Read the model definition and answer for the solid it produces. Units are mm, in the model's axes. A direction names the side the tool comes from. Coordinates: 2 decimals unless noted, no trailing zeros. Loops run counter-clockwise (first coordinate to the right, second up) from the corner with the lowest first, then second, coordinate; pieces in that order, holes last.
from build123d import *

# Parameters (mm, degrees)
SKETCH1_W                 = 201.168
SKETCH1_H                 = 201.168
BOSS_EXTRUDE1_DEPTH       = 1.5875
CUT_EXTRUDE1_REACH        = 144.256
SKETCH2_R                 = 16.5
F_1_4_CLEARANCE_HOLE1_D   = 6.7564
CHAMFER1_SIZE             = 6.35
CUT_EXTRUDE3_REACH        = 144.256
CUT_EXTRUDE4_REACH        = 144.256
CUT_EXTRUDE5_REACH        = 144.256
SKETCH7_W                 = 6.7564
SKETCH7_H                 = 14.478
SKETCH7_W_2               = 14.478
SKETCH7_H_2               = 6.7564
PORT_FOR_POWER_PLUG_REACH = 144.256
SKETCH8_R                 = 6.35


with BuildPart() as part:
    # Sketch1 → Boss-Extrude1 (new body)
    with BuildSketch(Plane.XY):
        Rectangle(SKETCH1_W, SKETCH1_H)
    extrude(amount=BOSS_EXTRUDE1_DEPTH)

    # Sketch2 → Cut-Extrude1 (cut, up to next)
    with BuildSketch(Plane.XY.offset(1.5875), mode=Mode.PRIVATE) as cut_extrude1_sk1:
        with Locations((-49.784, -40.5765)):
            Circle(SKETCH2_R)
    cut_extrude1_tool1 = extrude(cut_extrude1_sk1.sketch, amount=-CUT_EXTRUDE1_REACH, mode=Mode.PRIVATE) & part.part
    # Sketch2 → Cut-Extrude1 (cut, up to next)
    with BuildSketch(Plane.XY.offset(1.5875), mode=Mode.PRIVATE) as cut_extrude1_sk2:
        with Locations((39.4206, -52.284)):
            Circle(SKETCH2_R)
    cut_extrude1_tool2 = extrude(cut_extrude1_sk2.sketch, amount=-CUT_EXTRUDE1_REACH, mode=Mode.PRIVATE) & part.part
    add(cut_extrude1_tool1.solids().sort_by_distance((-49.784, -40.5765, 1.5875))[0], mode=Mode.SUBTRACT)
    add(cut_extrude1_tool2.solids().sort_by_distance((39.4206, -52.284, 1.5875))[0], mode=Mode.SUBTRACT)

    # 1/4 Clearance Hole1 (through all)
    with Locations(Plane.XY.offset(1.5875)):
        with Locations((-57.94375, 87.884), (57.94375, 87.884), (87.884, 0), (-87.884, 0), (-60.325, -87.884), (60.325, -87.884)):
            Hole(F_1_4_CLEARANCE_HOLE1_D / 2)

    # Chamfer1
    chamfer1_edges = [part.edges().sort_by_distance(p)[0] for p in [
        (100.584, -100.584, 0.79375),
        (-100.584, -100.584, 0.79375),
        (-100.584, 100.584, 0.79375),
        (100.584, 100.584, 0.79375),
    ]]
    chamfer(chamfer1_edges, length=CHAMFER1_SIZE)

    # Sketch5 → Cut-Extrude3 (cut, up to next)
    with BuildSketch(Plane(origin=(0, 0, 0), x_dir=(-1, 0, 0), z_dir=(0, 0, -1)), mode=Mode.PRIVATE) as cut_extrude3_sk1:
        with BuildLine():
            Line((33.284, -40.5765), (33.284, -71.0565))
            Line((33.284, -71.0565), (66.284, -71.0565))
            Line((66.284, -71.0565), (66.284, -40.5765))
            ThreePointArc((66.284, -40.5765), (49.784, -57.0765), (33.284, -40.5765))
        make_face()
    cut_extrude3_tool1 = extrude(cut_extrude3_sk1.sketch, amount=-CUT_EXTRUDE3_REACH, mode=Mode.PRIVATE) & part.part
    add(cut_extrude3_tool1.solids().sort_by_distance((-49.784, -61.908997, 0))[0], mode=Mode.SUBTRACT)

    # Sketch6 → Cut-Extrude4 (cut, up to next)
    with BuildSketch(Plane(origin=(0, 0, 0), x_dir=(-1, 0, 0), z_dir=(0, 0, -1)), mode=Mode.PRIVATE) as cut_extrude4_sk1:
        with BuildLine():
            Line((-50.165, 49.768115066), (-50.165, 51.308))
            ThreePointArc((-50.165, 51.308), (-50.8, 51.943), (-51.435, 51.308))
            Line((-51.435, 51.308), (-51.435, 49.768115066))
            ThreePointArc((-51.435, 49.768115066), (-50.8, 24.384), (-50.165, 49.768115066))
        make_face()
    cut_extrude4_tool1 = extrude(cut_extrude4_sk1.sketch, amount=-CUT_EXTRUDE4_REACH, mode=Mode.PRIVATE) & part.part
    # Sketch6 → Cut-Extrude4 (cut, up to next)
    with BuildSketch(Plane(origin=(0, 0, 0), x_dir=(-1, 0, 0), z_dir=(0, 0, -1)), mode=Mode.PRIVATE) as cut_extrude4_sk2:
        with BuildLine():
            Line((51.435, 49.768115066), (51.435, 51.308))
            ThreePointArc((51.435, 51.308), (50.8, 51.943), (50.165, 51.308))
            Line((50.165, 51.308), (50.165, 49.768115066))
            ThreePointArc((50.165, 49.768115066), (50.8, 24.384), (51.435, 49.768115066))
        make_face()
    cut_extrude4_tool2 = extrude(cut_extrude4_sk2.sketch, amount=-CUT_EXTRUDE4_REACH, mode=Mode.PRIVATE) & part.part
    add(cut_extrude4_tool1.solids().sort_by_distance((50.8, 37.153354, 0))[0], mode=Mode.SUBTRACT)
    add(cut_extrude4_tool2.solids().sort_by_distance((-50.8, 37.153354, 0))[0], mode=Mode.SUBTRACT)

    # Sketch7 → Cut-Extrude5 (cut, up to next)
    with BuildSketch(Plane(origin=(0, 0, 0), x_dir=(-1, 0, 0), z_dir=(0, 0, -1)), mode=Mode.PRIVATE) as cut_extrude5_sk1:
        with Locations((-57.94375, 95.123)):
            Rectangle(SKETCH7_W, SKETCH7_H)
    cut_extrude5_tool1 = extrude(cut_extrude5_sk1.sketch, amount=-CUT_EXTRUDE5_REACH, mode=Mode.PRIVATE) & part.part
    # Sketch7 → Cut-Extrude5 (cut, up to next)
    with BuildSketch(Plane(origin=(0, 0, 0), x_dir=(-1, 0, 0), z_dir=(0, 0, -1)), mode=Mode.PRIVATE) as cut_extrude5_sk2:
        with Locations((57.94375, 95.123)):
            Rectangle(SKETCH7_W, SKETCH7_H)
    cut_extrude5_tool2 = extrude(cut_extrude5_sk2.sketch, amount=-CUT_EXTRUDE5_REACH, mode=Mode.PRIVATE) & part.part
    # Sketch7 → Cut-Extrude5 (cut, up to next)
    with BuildSketch(Plane(origin=(0, 0, 0), x_dir=(-1, 0, 0), z_dir=(0, 0, -1)), mode=Mode.PRIVATE) as cut_extrude5_sk3:
        with Locations((95.123, 0)):
            Rectangle(SKETCH7_W_2, SKETCH7_H_2)
    cut_extrude5_tool3 = extrude(cut_extrude5_sk3.sketch, amount=-CUT_EXTRUDE5_REACH, mode=Mode.PRIVATE) & part.part
    # Sketch7 → Cut-Extrude5 (cut, up to next)
    with BuildSketch(Plane(origin=(0, 0, 0), x_dir=(-1, 0, 0), z_dir=(0, 0, -1)), mode=Mode.PRIVATE) as cut_extrude5_sk4:
        with Locations((60.325, -95.123)):
            Rectangle(SKETCH7_W, SKETCH7_H)
    cut_extrude5_tool4 = extrude(cut_extrude5_sk4.sketch, amount=-CUT_EXTRUDE5_REACH, mode=Mode.PRIVATE) & part.part
    # Sketch7 → Cut-Extrude5 (cut, up to next)
    with BuildSketch(Plane(origin=(0, 0, 0), x_dir=(-1, 0, 0), z_dir=(0, 0, -1)), mode=Mode.PRIVATE) as cut_extrude5_sk5:
        with Locations((-60.325, -95.123)):
            Rectangle(SKETCH7_W, SKETCH7_H)
    cut_extrude5_tool5 = extrude(cut_extrude5_sk5.sketch, amount=-CUT_EXTRUDE5_REACH, mode=Mode.PRIVATE) & part.part
    # Sketch7 → Cut-Extrude5 (cut, up to next)
    with BuildSketch(Plane(origin=(0, 0, 0), x_dir=(-1, 0, 0), z_dir=(0, 0, -1)), mode=Mode.PRIVATE) as cut_extrude5_sk6:
        with Locations((-95.123, 0)):
            Rectangle(SKETCH7_W_2, SKETCH7_H_2)
    cut_extrude5_tool6 = extrude(cut_extrude5_sk6.sketch, amount=-CUT_EXTRUDE5_REACH, mode=Mode.PRIVATE) & part.part
    add(cut_extrude5_tool1.solids().sort_by_distance((57.94375, 95.123, 0))[0], mode=Mode.SUBTRACT)
    add(cut_extrude5_tool2.solids().sort_by_distance((-57.94375, 95.123, 0))[0], mode=Mode.SUBTRACT)
    add(cut_extrude5_tool3.solids().sort_by_distance((-95.123, 0, 0))[0], mode=Mode.SUBTRACT)
    add(cut_extrude5_tool4.solids().sort_by_distance((-60.325, -95.123, 0))[0], mode=Mode.SUBTRACT)
    add(cut_extrude5_tool5.solids().sort_by_distance((60.325, -95.123, 0))[0], mode=Mode.SUBTRACT)
    add(cut_extrude5_tool6.solids().sort_by_distance((95.123, 0, 0))[0], mode=Mode.SUBTRACT)

    # Sketch8 → PORT FOR POWER PLUG (cut, up to next)
    with BuildSketch(Plane(origin=(0, 0, 0), x_dir=(-1, 0, 0), z_dir=(0, 0, -1)), mode=Mode.PRIVATE) as port_for_power_plug_sk1:
        with Locations((-1.533105196, -45.535092969)):
            Circle(SKETCH8_R)
    port_for_power_plug_tool1 = extrude(port_for_power_plug_sk1.sketch, amount=-PORT_FOR_POWER_PLUG_REACH, mode=Mode.PRIVATE) & part.part
    add(port_for_power_plug_tool1.solids().sort_by_distance((1.533105, -45.535093, 0))[0], mode=Mode.SUBTRACT)


solid = part.part
Item 1: Determine the mould class of faces 1 (the face through (51.35, 24.396, 0.783)), 2 (the face through (-1, 1, 0)), 3 (the face through (97.453, 97.365, 0.783)) for opening direction X: released by +X, released by -X, zero draft, split by the parting line, or undercut.
Numbers:
face 1: undercut
face 2: zero draft
face 3: released by +X
Item 2: Find the intervals of material crossed by line 1 along X through (y, z) = (91, 0.4); line 2 along Y through (x, z) = (50.8, 0.5); line 3 along X through (y, z) = (32, 0.15), in increasing order.
Numbers:
line 1: x = -100.58 to -61.32, -54.57 to 54.57, 61.32 to 100.58
line 2: y = -100.58 to -64.23, -40.34 to 24.38, 51.94 to 100.58
line 3: x = -100.58 to -62.44, -39.16 to 39.16, 62.44 to 100.58
Item 3: A cutting plane is placed at A-A on x = 2.5. Determine the outline of the cut face in (y, z).
Numbers:
outline: (-100.58, 0) - (-51.81, 0) - (-51.81, 1.59) - (-100.58, 1.59) - close; (-39.26, 0) - (100.58, 0) - (100.58, 1.59) - (-39.26, 1.59) - close
Item 4: A cutting plane is placed at B-B on x = -46. Determine the outline of the cut face in (y, z), then the cut area to 3 significant figures.
Numbers:
outline: (-100.58, 0) - (-71.06, 0) - (-71.06, 1.59) - (-100.58, 1.59) - close; (-24.52, 0) - (25.33, 0) - (25.33, 1.59) - (-24.52, 1.59) - close; (48.84, 0) - (100.58, 0) - (100.58, 1.59) - (48.84, 1.59) - close
area: 208 mm2
Item 5: Which of the six approach directions +Z, -Z, +X, -X, +Y, -Y give full straight-line access (tool end or side, diameter ignored) to faces 4 (the face through (-49.42, -24.08, 0.8)), 5 (the face through (97.453, -97.365, 0.783))?
Numbers:
face 4: +Z, -Z
face 5: +Z, -Z, +X, -Y
Item 6: A cutting plane is placed at D-D on y = 0. Determine the outline of the cut face in (x, z).
Numbers:
outline: (-84.51, 0) - (84.51, 0) - (84.51, 1.59) - (-84.51, 1.59) - close
Item 7: A cutting plane is placed at C-C on y = -56.5. Determine the outline of the cut face in (x, z).
Numbers:
outline: (-100.58, 0) - (-66.28, 0) - (-66.28, 1.59) - (-100.58, 1.59) - close; (-33.28, 0) - (23.47, 0) - (23.47, 1.59) - (-33.28, 1.59) - close; (55.37, 0) - (100.58, 0) - (100.58, 1.59) - (55.37, 1.59) - close
